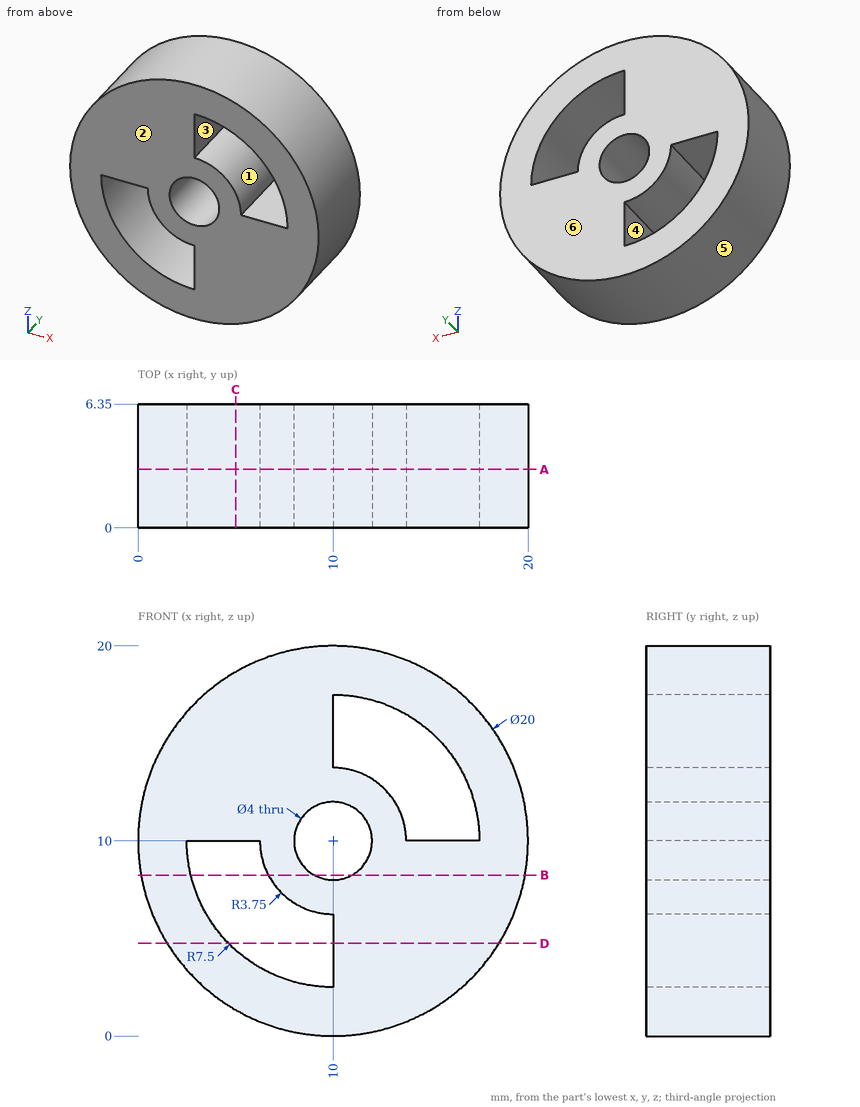
The drawing under review shows one solid part. Ordinate dimensions are in mm from its lowest x, y, z. A direction names the side the tool comes from. Coordinates: 2 decimals unless noted, no trailing zeros. Order: outer loops, then holes, each group sorted by start corner. A loop starts at its lowest first (then second) coordinate and runs counter-clockwise, first axis right, second up. Notation, with made-up numbers: (-2.75, 42.25) -> (20.25, 42.25) arc R20 cw to (20.25, 53.25) -> close; hole circle Ø8 at (20, 76.5). An arc over 180 degrees is marked (long way). Answer in a Markdown table with one row per item. Add a question column.
Item 1: Machinability: for the marked faces 1 and 2, which of the approach directions +Z, -Z, +X, -X, +Y, -Y give a long, thin tool a straight path to every point of the face, cutting with its end or side? Answer none if there is none.
Item 2: We need section D-D on z = 4.75. Write out the cut boundary in (x, y), plus the area to 3 significant figures.
Item 3: We need section A-A on y = 3. Write out the cut boundary in (x, z).
Item 4: We need section C-C on x = 5. Write out the cut boundary in (y, z), plus the area to 3 significant figures.
Item 5: We need section B-B on z = 8.25. Write out the cut boundary in (x, y), plus the area to 3 significant figures.
Item 6: Clearance check with flat-ended pins moving along their axes: pin 1 (8 mm diameter, centred on x = 7.5, z = 9, fed in from -Y); pin 2 (1.9 mm diameter, centred on x = 3.5, y = 3.5, fed in from -Z); pin 3 (3 mm diameter, centred on y = 3, z = 15.5, fed in from +X); pin 4 (1.5 mm diameter, centred on y = 4, z = 7, fed in from +X). State where each tip first meets the part, or that it passes through.
Item 7: Mouldability with a two-part tool opening along Z and no side actions: class the marked faces 3, 4, 5 and 6 as +Z half, -Z half, draft (parallel to the pull), parting line (faces both ways), or undercut.
Item 8: To check wall thickness, follow probe 1 along Z at (x, y) = (10.75, 4.75); probe 2 along Z at (x, y) = (15.5, 4.25); probe 3 along X at (y, z) = (1, 8.5). State the ranges of each line that lie inside material, in increasing order.
Final values:
| question | item | result |
|---|---|---|
| 1 | face 1 | +Y, -Y |
| 1 | face 2 | +Z, -Z, +X, -X, -Y |
| 2 | outline | (1.49, 0) -> (4.64, 0) -> (4.64, 6.35) -> (1.49, 6.35) -> close; (10, 0) -> (18.51, 0) -> (18.51, 6.35) -> (10, 6.35) -> close |
| 2 | area | 74.1 mm2 |
| 3 | outline | circle Ø20 at (10, 10); hole (2.5, 10) arc R7.5 ccw to (10, 2.5) -> (10, 6.25) arc R3.75 cw to (6.25, 10) -> close; hole circle Ø4 at (10, 10); hole (10, 13.75) arc R3.75 cw to (13.75, 10) -> (17.5, 10) arc R7.5 ccw to (10, 17.5) -> close |
| 4 | outline | (0, 1.34) -> (6.35, 1.34) -> (6.35, 4.41) -> (0, 4.41) -> close; (0, 10) -> (6.35, 10) -> (6.35, 18.66) -> (0, 18.66) -> close |
| 4 | area | 74.5 mm2 |
| 5 | outline | (0.15, 0) -> (2.71, 0) -> (2.71, 6.35) -> (0.15, 6.35) -> close; (6.68, 0) -> (9.03, 0) -> (9.03, 6.35) -> (6.68, 6.35) -> close; (10.97, 0) -> (19.85, 0) -> (19.85, 6.35) -> (10.97, 6.35) -> close |
| 5 | area | 87.5 mm2 |
| 6 | pin 1 | stops at y = 0 |
| 6 | pin 2 | stops at z = 1.68 |
| 6 | pin 3 | stops at x = 19.17 |
| 6 | pin 4 | stops at x = 19.74 |
| 7 | face 3 | undercut |
| 7 | face 4 | undercut |
| 7 | face 5 | parting line |
| 7 | face 6 | draft |
| 8 | probe 1 | z = 0.03 to 8.15, 11.85 to 13.67, 17.46 to 19.97 |
| 8 | probe 2 | z = 1.65 to 10, 15.1 to 18.35 |
| 8 | probe 3 | x = 0.11 to 2.65, 6.56 to 8.68, 11.32 to 19.89 |
